Geometry: final body of the model. Coordinates: model frame, mm. A direction names the side the tool comes from. Give positions to 0.01 mm unless a question says otherwise; leave off trailing zeros. Write each loop counter-clockwise with the first axis right and the second up, starting at its lowest first coordinate (ties: lowest second). Pieces come first, ordered by that corner, then holes. Notation, with made-up numbers: M 25.25,-34 L 84.25,-34 A25 cw 84.25,-9 Z; hole C 55,34.25 d10. An arc over 180 degrees is marked long. Use a Markdown table: item, result. Add a question column.
(1) Draft query along Y for faces 4 (the cylindrical face through (54.705, 1.933, 42.818)), 5 (the cylindrical face through (-51.73, 21.45, -2.96)), 6 (the cylindrical face through (13.93, 58.39, 52.58)). Return one class per face: released by +Y, released by -Y, zero draft, split by the parting line, or undercut.
(2) Reachability of faces 1 (the flat face through (-9, 47, 37)), 2 (the flat face through (14, 62, 34)), 3 (the flat face through (-34.61, 21.7, 40.28)) from +Z, -Z, +X, -X, +Y, -Y: full face, straight path, thin tool, end or side. Return the list, or none.
(3) Cut plane C-C (z = 17.5). Output: boundary loops of the cut face in (x, y), plus the area to 3 significant figures.
(4) Cut plane B-B (y = 59). Output: boundary loops of the cut face in (x, z).
(5) Cut plane D-D (x = 0). Output: boundary loops of the cut face in (y, z).
(6) Cut plane A-A (z = 36). Output: boundary loops of the cut face in (x, y), plus the area to 3 significant figures.
(7) Pin query (flat end, axial travel): pin 1 Ø5 at (x, z) = (-53.5, 34.5) entering from +Y; pin 2 Ø2 at (x, y) = (-29, -52.5) entering from +Z; pin 3 Ø11.5 at (y, z) = (50, 44) entering from +X. Return the tip coordinate at first contact, or that it passes through.
(8) Material intervals for L1, parallel to Y at x = 15.5, z = 44; L2, parallel to Y at x = 50.5, z = 1; L3, parallel to X at y = -51, z = 20, sorted ascending.
Autodesk Inventor part; units mm, degrees
ref_plane "YZ Plane" through (0, 0, 0) normal (1, 0, 0) x (0, 1, 0)
ref_plane "XZ Plane" through (0, 0, 0) normal (0, 1, 0) x (-1, 0, 0)
ref_plane "XY Plane" through (0, 0, 0) normal (0, 0, 1) x (1, 0, 0)
sketch "Sketch1" plane through (0, 0, 0) normal (0, 0, 1) x (1, 0, 0)
  line L0 (-51, 77) -> (51, 77)
  line L1 (77, 51) -> (77, -51)
  line L2 (51, -77) -> (-51, -77)
  line L3 (-77, -51) -> (-77, 51)
  line L4 (-77, 77) -> (77, -77) construction
  line L5 (77, 77) -> (-77, -77) construction
  arc A0 (-51, 77) -> (-77, 51) centre (-51, 51) ccw
  arc A1 (-77, -51) -> (-51, -77) centre (-51, -51) ccw
  arc A2 (51, -77) -> (77, -51) centre (51, -51) ccw
  arc A3 (77, 51) -> (51, 77) centre (51, 51) ccw
  point P0 (0, 0)
  dimension "d0" = 154
  dimension "d1" = 154
  dimension "d2" = 26
extrude "Extrusion1" add sketch "Sketch1" along normal blind 25
sketch "Sketch2" plane through (0, 0, 25) normal (0, 0, 1) x (1, 0, 0)
  arc A0 (-77, -51) -> (-51, -77) centre (-51, -51) ccw
  arc A1 (51, -77) -> (77, -51) centre (51, -51) ccw
  arc A2 (77, 51) -> (51, 77) centre (51, 51) ccw
  arc A3 (-51, 77) -> (-77, 51) centre (-51, 51) ccw
  point P0 (0, 0)
hole "Hole1" at (-51, -51, 25) at (51, -51, 25) at (51, 51, 25) at (-51, 51, 25) direction (0, 0, -1) diameter 20 end through all
sketch "Sketch3" plane through (0, 0, 0) normal (0, 0, -1) x (-1, 0, 0)
  circle A0 centre (0, 0) radius 56
  dimension "d12" = 112
extrude "Extrusion2" add sketch "Sketch3" along normal blind 6
sketch "Sketch4" plane through (0, 0, 25) normal (0, 0, 1) x (1, 0, 0)
  line L0 (51, 77) -> (-51, 77)
sketch "Sketch5" plane through (0, 0, 25) normal (0, 0, 1) x (1, 0, 0)
  arc A0 (50.6713, -17.3833) -> (50.6713, 17.3833) centre (46, 0) ccw
  arc A1 (-50.6713, 17.3833) -> (-50.6713, -17.3833) centre (-46, 0) ccw
  line L0 (0, 31) -> (0, -31) construction
  line L1 (19, 62) -> (-19, -62) construction
  line L2 (-19, 62) -> (19, -62) construction
  line L3 (-9, 62) -> (-9, 31)
  line L4 (-9, 31) -> (9, 31)
  line L5 (9, 31) -> (9, 62)
  line L6 (-9, -62) -> (-9, -31)
  line L7 (-9, -31) -> (9, -31)
  line L8 (9, -31) -> (9, -62)
  line L9 (19, 62) -> (9, 62)
  line L10 (-9, 62) -> (-19, 62)
  line L11 (-19, -62) -> (-9, -62)
  line L12 (9, -62) -> (19, -62)
  line L13 (19, -62) -> (19, -25.8942)
  line L14 (19, 25.8942) -> (19, 62)
  line L15 (-19, 62) -> (-19, 25.8942)
  line L16 (-19, -25.8942) -> (-19, -62)
  line L17 (-19, 25.8942) -> (-50.6713, 17.3833)
  line L18 (-19, -25.8942) -> (-50.6713, -17.3833)
  line L19 (50.6713, -17.3833) -> (19, -25.8942)
  line L20 (50.6713, 17.3833) -> (19, 25.8942)
  point P0 (0, 0)
  dimension "d34" = 36
  dimension "d35" = 36
  dimension "d36" = 92
  dimension "d37" = 46
  dimension "d38" = 62
  dimension "d41" = 38
  dimension "d42" = 124
  dimension "d43" = 18
  dimension "d44" = 31
  dimension "d46" = 18
  dimension "d47" = 31
extrude "Extrusion3" add sketch "Sketch5" along normal blind 31
sketch "Sketch6" plane through (0, 0, 56) normal (0, 0, 1) x (1, 0, 0)
  arc A0 (-50.6713, 17.3833) -> (-50.6713, -17.3833) centre (-46, 0) ccw
  arc A1 (50.6713, -17.3833) -> (50.6713, 17.3833) centre (46, 0) ccw
  point P0 (0, 0)
hole "Hole2" at (-46, 0, 56) at (46, 0, 56) direction (0, 0, -1) diameter 17.8349 depth 26 tip angle 118
fillet "Fillet1" radius 12 4 edges at (-14, -62, 56) (14, -62, 56) (14, 62, 56) (-14, 62, 56)
sketch "Sketch7" plane through (-19, -62, 25) normal (-1, 0, 0) x (0, 0, 1)
  arc A0 (19, 0) -> (31, 12) centre (19, 12) ccw
  arc A1 (31, 112) -> (19, 124) centre (19, 112) ccw
  point P0 (-25, 62)
hole "Hole3" at (-19, -50, 44) at (-19, 50, 44) direction (1, 0, 0) diameter 10 end through all
properties part number "cad@74"
Answer list:
| question | item | result |
|---|---|---|
| 1 | face 4 | undercut |
| 1 | face 5 | split by the parting line |
| 1 | face 6 | released by +Y |
| 2 | face 1 | +Z, +Y |
| 2 | face 2 | +Z, +X, -X, +Y |
| 2 | face 3 | +Z, -X, +Y |
| 3 | outline | M -77,-51 A26 ccw -51,-77 L 51,-77 A26 ccw 77,-51 L 77,51 A26 ccw 51,77 L -51,77 A26 ccw -77,51 Z; hole C -51,-51 d20; hole C -51,51 d20; hole C 51,-51 d20; hole C 51,51 d20 |
| 3 | area | 21,900 mm² |
| 4 | outline | M -75.74,0 L -57,0 L -57,25 L -75.74,25 Z; M -45,0 L 45,0 L 45,25 L 19,25 L 19,51.94 L 9,51.94 L 9,25 L -9,25 L -9,51.94 L -19,51.94 L -19,25 L -45,25 Z; M 57,0 L 75.74,0 L 75.74,25 L 57,25 Z |
| 5 | outline | M -77,0 L -56,0 L -56,-6 L 56,-6 L 56,0 L 77,0 L 77,25 L 31,25 L 31,56 L -31,56 L -31,25 L -77,25 Z |
| 6 | outline | M -50.67,-17.38 L -19,-25.89 L -19,-62 L -9,-62 L -9,-31 L 9,-31 L 9,-62 L 19,-62 L 19,-25.89 L 50.67,-17.38 A18 ccw 50.67,17.38 L 19,25.89 L 19,62 L 9,62 L 9,31 L -9,31 L -9,62 L -19,62 L -19,25.89 L -50.67,17.38 A18 ccw Z; hole C -46,0 d17.83; hole C 46,0 d17.83 |
| 6 | area | 6,520 mm² |
| 7 | pin 1 | y = 17.29 |
| 7 | pin 2 | z = 25 |
| 7 | pin 3 | x = 19 |
| 8 | L1 | -62 to -55, -45 to 45, 55 to 62 |
| 8 | L2 | -77 to -60.99, -41.01 to 41.01, 60.99 to 77 |
| 8 | L3 | -77 to -61, -41 to 41, 61 to 77 |
